```python
from build123d import *

# Parameters (mm, degrees)
SKETCH1_W           = 250
SKETCH1_H           = 100
BOSS_EXTRUDE1_DEPTH = 10
SKETCH2_R           = 5
BOSS_EXTRUDE2_DEPTH = 30
SKETCH3_W           = 250
SKETCH3_H           = 100
BOSS_EXTRUDE3_DEPTH = 10
SKETCH5_W           = 50
SKETCH5_H           = 50
CUT_EXTRUDE1_DEPTH  = 10
FILLET1_R           = 5


with BuildPart() as part:
    # Sketch1 → Boss-Extrude1 (new body)
    with BuildSketch(Plane.XY):
        Rectangle(SKETCH1_W, SKETCH1_H)
    extrude(amount=BOSS_EXTRUDE1_DEPTH)

    # Sketch2 → Boss-Extrude2 (add)
    with BuildSketch(Plane.XY.offset(10)):
        with Locations((75, 0)):
            Circle(SKETCH2_R)
        with Locations((-25, 0)):
            Circle(SKETCH2_R)
    extrude(amount=BOSS_EXTRUDE2_DEPTH)

    # Sketch3 → Boss-Extrude3 (add)
    with BuildSketch(Plane.XY.offset(40)):
        Rectangle(SKETCH3_W, SKETCH3_H)
    extrude(amount=BOSS_EXTRUDE3_DEPTH)

    # Sketch5 → Cut-Extrude1 (cut)
    with BuildSketch(Plane(origin=(0, 0, 0), x_dir=(-1, 0, 0), z_dir=(0, 0, -1))):
        with Locations((95, 0)):
            Rectangle(SKETCH5_W, SKETCH5_H)
    extrude(amount=-CUT_EXTRUDE1_DEPTH, mode=Mode.SUBTRACT)

    # Fillet1
    fillet1_edges = [part.edges().sort_by_distance(p)[0] for p in [
        (-120, 25, 5),
        (-120, -25, 5),
        (-70, -25, 5),
        (-70, 25, 5),
    ]]
    fillet(fillet1_edges, radius=FILLET1_R)


solid = part.part
```
Read the model definition and answer for the solid it produces. Units are mm, in the model's axes. A direction names the side the tool comes from. Coordinates: 2 decimals unless noted, no trailing zeros. Order: outer loops, then holes, each group sorted by start corner. A loop starts at its lowest first (then second) coordinate and runs counter-clockwise, first axis right, second up. Notation, with made-up numbers: (80.25, 86) - (107.25, 86) arc R21 ccw to (107.25, 105) - close; hole circle Ø5 at (6, 18). An arc over 180 degrees is marked (long way). Answer as a JSON object with one key per item and string values. Group by question number.
Item 1: Section A-A (y = 0) is taken. Give the vertices of the cut face in (x, z).
Item 2: Section C-C (y = 33) is taken. Give the vertices of the cut face in (x, z).
Item 3: Flat-ended cylindrical pins translate along their axes: P1, Ø1.5, axis at x = 45, y = -21, coming from the -Z side; P2, Ø6, axis at x = -16.5, z = 22, coming from the +Y side; P3, Ø6, axis at x = -27.5, z = 33.5, coming from the +Y side. Find the tip coordinate at first contact, or state that the pin passes through.
Item 4: Consider probe 1 along X at (y, z) = (16, 8.5); probe 2 along Z at (x, y) = (-68.5, 19); probe 3 along Y at (x, z) = (73.5, 29). Determine where each line is inside the solid, lowest interval first. Write a range as from..to.
Item 5: A tool of negligible diameter and unlimited length cuts with its end or side. For faces 4 (the face through (125, -1, 5)), 5 (the face through (79.619, -1.915, 24.79)), 6 (the face through (-95, -25, 5)), from which of +Z, -Z, +X, -X, +Y, -Y can it reach the whole face along a straight path? Write none if from no direction.
Item 6: Section D-D (x = -104) is taken. Give the vertices of the cut face in (y, z).
Item 7: Section B-B (x = -65) is taken. Give the vertices of the cut face in (y, z), plus the area to 3 significant figures.
Item 8: The mould has two halves that part along Y. Classify faces 1 (the face through (-125, -1, 5)), 2 (the face through (-30, 0, 25)), 3 (the face through (-120, 0, 5)): +Y half, -Y half, draft (parallel to the pull), parting line (faces both ways), or undercut.
Results are:
{
 "1": {"outline": "(-125, 0) - (-120, 0) - (-120, 10) - (-125, 10) - close; (-125, 40) - (-30, 40) - (-30, 10) - (-70, 10) - (-70, 0) - (125, 0) - (125, 10) - (80, 10) - (80, 40) - (125, 40) - (125, 50) - (-125, 50) - close; hole (-20, 10) - (70, 10) - (70, 40) - (-20, 40) - close"},
 "2": {"outline": "(-125, 0) - (125, 0) - (125, 10) - (-125, 10) - close; (-125, 40) - (125, 40) - (125, 50) - (-125, 50) - close"},
 "3": {"P1": "stops at z = 0", "P2": "passes through", "P3": "stops at y = 5"},
 "4": {"probe 1": "x = -125..-120, -70..125", "probe 2": "z = 0..10, 40..50", "probe 3": "y = -4.77..4.77"},
 "5": {"face 4": "+Z, -Z, +X, +Y, -Y", "face 5": "none", "face 6": "-Z"},
 "6": {"outline": "(-50, 0) - (-25, 0) - (-25, 10) - (-50, 10) - close; (-50, 40) - (50, 40) - (50, 50) - (-50, 50) - close; (25, 0) - (50, 0) - (50, 10) - (25, 10) - close"},
 "7": {"outline": "(-50, 0) - (50, 0) - (50, 10) - (-50, 10) - close; (-50, 40) - (50, 40) - (50, 50) - (-50, 50) - close", "area": "2,000 mm^2"},
 "8": {"face 1": "draft", "face 2": "parting line", "face 3": "undercut"}
}
